```python
from build123d import *

# Parameters (mm, degrees)
F0_R     = 12
F1_DEPTH = 10
F2_R     = 10
F3_DEPTH = 33
F4_DEPTH = 54
F5_R     = 9
F6_DEPTH = 18
F9_DEPTH = 5.501
F10_SIZE = 1
F11_W    = 2.5
F11_H    = 0.980663


with BuildPart() as f1:
    # F0 (on Right) → F1 (new body)
    with BuildSketch(Plane.YZ):
        Circle(F0_R)
    extrude(amount=F1_DEPTH)

    # F2 (on face) → F3 (join)
    with BuildSketch(Plane(origin=(0, 0, 0), x_dir=(0, -1, 0), z_dir=(-1, 0, 0))):
        Circle(F2_R)
    extrude(amount=F3_DEPTH)

    # F2 (on face) → F4 (join)
    with BuildSketch(Plane(origin=(0, 0, 0), x_dir=(0, -1, 0), z_dir=(-1, 0, 0))):
        Circle(F2_R)
    extrude(amount=-F4_DEPTH)

    # F5 (on face) → F6 (join)
    with BuildSketch(Plane.YZ.offset(54)):
        Circle(F5_R)
    extrude(amount=F6_DEPTH)

    # F8 (on offset) → F9 (cut, through all)
    with BuildSketch(Plane.XZ.offset(-6.5)):
        with BuildLine():
            Line((-33, 3), (-33, -3))
            Line((-33, -3), (-6, -3))
            ThreePointArc((-6, -3), (-3, 0), (-6, 3))
            Line((-6, 3), (-33, 3))
        make_face()
    extrude(amount=-F9_DEPTH, mode=Mode.SUBTRACT)

    # F10
    f10_edges = [f1.edges().sort_by_distance(p)[0] for p in [
        (-33, -1.517577, -9.884177),
        (-33, -1.517577, 9.884177),
        (72, -9, 0),
    ]]
    chamfer(f10_edges, length=F10_SIZE)

    # F11 (on Top) → F12 (revolve, cut)
    with BuildSketch(Plane.XY):
        with Locations((61.25, 9.490331)):
            Rectangle(F11_W, F11_H)
        Polygon((62.5, 9), (60, 9), (60, -9), (62.8, -9), align=None)
        Polygon((62.8, -9), (60, -9), (60, -10.015493), (62.816925, -10.015493), align=None)
    revolve(axis=Axis((60, -0.455183, 0), (0, -1, 0)), mode=Mode.SUBTRACT)


solid = f1.part
```
Read the model definition and answer for the solid it produces. Units are mm, in the model's axes. A direction names the side the tool comes from. Give positions to 0.01 mm unless a question says otherwise; leave off trailing zeros. Loops run counter-clockwise (first coordinate to the right, second up) from the corner with the lowest first, then second, coordinate; pieces in that order, holes last.
Item 1: The part is cut by section D-D (x = 13.5). Write down the section's boundary in (y, z), and give its area (3 significant figures).
Item 2: The part is cut by section B-B (x = 1). Write down the section's boundary in (y, z).
Item 3: Find the intervals of material crossed by line 1 along X through (y, z) = (5.25, -9.5); line 2 along X through (y, z) = (7.75, -1.75); line 3 along Z through (x, y) = (52.5, -6), in increasing order.
Item 4: The part is cut by section A-A (y = 0). Write down the section's boundary in (x, z).
Item 5: Each of these flat-tipped pins is pushed along its axis until it touches: pin 1 Ø3 at (x, y) = (-16.5, 5) entering from -Z; pin 2 Ø3.5 at (x, y) = (-15.5, 8.5) entering from -Z; pin 3 Ø3 at (x, z) = (25.5, -4) entering from +Y; pin 4 Ø4 at (x, z) = (6, 1) entering from +Y. Where does it stop, or does it pass through?
Item 6: The mould has two halves that part along Z. Classify faces 1 (the flat face through (0, -5, 9)), 2 (the conical face through (-32.84, -9.152, -0.364)), 3 (the flat face through (-19, 8, 3)), 4 (the flat face through (-20, 8, -3)): released by +Z, released by -Z, zero draft, split by the parting line, or undercut.
Item 7: The part is cut by section C-C (x = -20). Write down the section's boundary in (y, z), and give its area (3 significant figures).
Item 8: For faces 5 (the cylindrical face through (31.69, 2.17, -9.76)), 6 (the cylindrical face through (-3, 8, 0)), 7 (the cylindrical face through (-15.78, -9.54, 3)), determine the directions among +Z, -Z, +X, -X, +Y, -Y from which every point of the face is accessible in a straight line to the end or side of a thin tool.
Taken from the geometry:
1. outline: circle Ø20 at (0, 0)
1. area: 314 mm2
2. outline: circle Ø24 at (0, 0)
3. line 1: x = 0 to 10
3. line 2: x = -3.56 to 58.19, 61.81 to 72
3. line 3: z = -8 to 8
4. outline: (-33, -9) - (-32, -10) - (0, -10) - (0, -12) - (10, -12) - (10, -10) - (54, -10) - (54, -9) - (71, -9) - (72, -8) - (72, 8) - (71, 9) - (54, 9) - (54, 10) - (10, 10) - (10, 12) - (0, 12) - (0, 10) - (-32, 10) - (-33, 9) - close; hole circle Ø5.3 at (60, 0)
5. pin 1: stops at z = -9.37
5. pin 2: stops at z = -7.38
5. pin 3: stops at y = 9.68
5. pin 4: stops at y = 12
6. face 1: zero draft
6. face 2: split by the parting line
6. face 3: undercut
6. face 4: undercut
7. outline: (6.5, -3) - (6.5, 3) - (9.54, 3) arc R10 ccw (long way) to (9.54, -3) - close
7. area: 294 mm2
8. face 5: +X
8. face 6: -X, +Y
8. face 7: -X
